Input: part model. Units: mm. Frame: model coordinates. A direction names the side the tool comes from. Round coordinates to 2 decimals unless told otherwise and drop trailing zeros. Write each loop counter-clockwise with the first axis right and the second up, starting at its lowest first coordinate (ties: lowest second). Pieces come first, ordered by that corner, then holes. Notation, with made-up numbers: (-28.5, 38) -> (7.5, 38) arc R14 ccw to (7.5, 61) -> close; hole circle Ø8 at (67.25, 74.25). An arc over 180 degrees is marked (long way). Write item = value, one per line.
```python
from build123d import *

# Parameters (mm, degrees)
SKETCH_2_R               = 1.5
CUT_EXTRUDE_3_DEPTH      = 10
PATTERN_CIRCULAR_2_COUNT = 20
SKETCH_3_R               = 4
CUT_EXTRUDE_4_DEPTH      = 23.085770306


with BuildPart() as part:
    # 草图1 → 旋转1 (revolve)
    with BuildSketch(Plane(origin=(0, 0, 0), x_dir=(0, 0, -1), z_dir=(1, 0, 0))):
        Polygon((0, 4.050451807), (0, 17.050451807), (-12.625, 17.050451807), (-12.625, 15.550451807), (-10.125, 15.550451807), (-10.125, 5.550451807), (-12.625, 5.550451807), (-12.625, 4.050451807), align=None)
    revolve(axis=Axis((0, 33.241716867, 0), (0, -1, 0)))

    # 草图2 → 切除-拉伸3 (cut)
    with BuildSketch(Plane.XZ.offset(-15.550451807)):
        with Locations((-10.043642365, 1.280965666)):
            Circle(SKETCH_2_R)
    cut_extrude_3 = extrude(amount=CUT_EXTRUDE_3_DEPTH, mode=Mode.SUBTRACT)

    # 阵列(圆周)2: 切除-拉伸3 ×20 about axis
    pattern_circular_2_axis = Axis((0, 0, 0), (0, 1, 0))
    for i in range(1, PATTERN_CIRCULAR_2_COUNT):
        add(cut_extrude_3.rotate(pattern_circular_2_axis, i * 360 / PATTERN_CIRCULAR_2_COUNT), mode=Mode.SUBTRACT)

    # 草图3 → 切除-拉伸4 (cut, through all)
    with BuildSketch(Plane.XZ.offset(-4.050451807)):
        with Locations(Location((0, 0, 0), (0, 0, 270))):
            Circle(SKETCH_3_R)
    extrude(amount=-CUT_EXTRUDE_4_DEPTH, mode=Mode.SUBTRACT)


solid = part.part
```
1) Access query for faces 1 (the face through (-3.905, 10.459, 0.867)), 2 (the face through (-6.3, 10.62, 5.89)). Directions: +Z, -Z, +X, -X, +Y, -Y. A direction counts if a zero-diameter tool reaches every point of the face in a straight line with its end or side. Return the directions, or none.
Solutions:
face_1 = +Y, -Y
face_2 = none
2) Line query: L1, parallel to Y at x = 9, z = 5; L2, parallel to Z at x = 9, y = 6.25; L3, parallel to X at y = 8.5, z = 0. Output: solid intervals per line, ascending. Write a range as from..to.
Solutions:
L1 = 4.05..5.55, 15.55..17.05
L2 = -2.83..-2.36, -0.2..0.72, 3.05..3.37
L3 = -9.26..-4, 4..9.26
3) Cut plane A-A (z = -1). Return the cut outline in (x, y).
Solutions:
outline = (-12.59, 4.05) -> (-3.87, 4.05) -> (-3.87, 17.05) -> (-12.59, 17.05) -> (-12.59, 15.55) -> (-8.74, 15.55) -> (-8.74, 5.55) -> (-12.59, 5.55) -> close; (3.87, 4.05) -> (12.59, 4.05) -> (12.59, 5.55) -> (8.57, 5.55) -> (8.57, 15.55) -> (12.59, 15.55) -> (12.59, 17.05) -> (3.87, 17.05) -> close
4) Cut plane B-B (x = 9). Return the cut outline in (y, z).
Solutions:
outline = (4.05, -8.85) -> (5.55, -8.85) -> (5.55, -2.83) -> (15.55, -2.83) -> (15.55, -8.85) -> (17.05, -8.85) -> (17.05, 8.85) -> (15.55, 8.85) -> (15.55, 3.37) -> (5.55, 3.37) -> (5.55, 8.85) -> (4.05, 8.85) -> close; hole (5.55, -2.36) -> (15.55, -2.36) -> (15.55, -0.2) -> (5.55, -0.2) -> close; hole (5.55, 0.72) -> (15.55, 0.72) -> (15.55, 3.05) -> (5.55, 3.05) -> close
5) Cut plane C-C (x = 1). Return the cut outline in (y, z).
Solutions:
outline = (4.05, -12.59) -> (5.55, -12.59) -> (5.55, -8.74) -> (15.55, -8.74) -> (15.55, -12.59) -> (17.05, -12.59) -> (17.05, -3.87) -> (4.05, -3.87) -> close; (4.05, 3.87) -> (17.05, 3.87) -> (17.05, 12.59) -> (15.55, 12.59) -> (15.55, 8.57) -> (5.55, 8.57) -> (5.55, 12.59) -> (4.05, 12.59) -> close
6) First-contact query: P1, Ø1.5, axis at x = 8.5, z = 10, coming from the +Y side; P2, Ø1, axis at y = 7, z = 2.5, coming from the +X side; P3, Ø1, axis at y = 9.5, z = 1.5, coming from the -X side; P4, Ø5, axis at x = 7.5, y = 11.5, coming from the -Z side. Flat tips, straight axial feed; report the tip coordinate or a pass-through.
Solutions:
P1 = 17.05
P2 = 8.94
P3 = -8.73
P4 = -8.06
7) Draft query along Z for faces 3 (the face through (12.325, 4.79, -2.737)), 4 (the face through (-8.47, 10.62, -1.64)), 5 (the face through (-3, 17.05, 3)). Return one class per face: +Z half, -Z half, draft (parallel to the pull), parting line (faces both ways), or undercut.
Solutions:
face_3 = parting line
face_4 = undercut
face_5 = draft
